Autodesk Fusion 360 part; units mm, degrees
sketch "Sketch1" plane through (0, 0, 0) normal (0, 0, 1) x (1, 0, 0)
  line L0 (-2.875, 0) -> (2.875, 0)
  line L1 (-5.375, 2.5) -> (5.375, 2.5)
  line L2 (-5.375, 2.5) -> (-2.875, 0)
  line L3 (5.375, 2.5) -> (2.875, 0)
  line L4 (0, 7.9451) -> (0, -6.0549)
  dimension "d1" = 5.75
  dimension "d2" = 10.75
  dimension "d3" = 2.5
extrude "Extrude1" add sketch "Sketch1" along normal blind 60
sketch "Sketch2" plane through (0, 0, 0) normal (0, 0, -1) x (-1, 0, 0)
  line L0 (2.875, 0) -> (5.375, 2.5)
  line L1 (5.375, 2.5) -> (-5.375, 2.5)
  line L2 (-5.375, 2.5) -> (-2.875, 0)
  line L3 (-2.875, 0) -> (2.875, 0)
  line L4 (-5.375, 2.5) -> (5.375, 2.5)
  line L5 (5.375, 2.5) -> (5.375, -3)
  line L6 (5.375, -3) -> (-5.375, -3)
  line L7 (-5.375, -3) -> (-5.375, 2.5)
  dimension "d6" = 10.75
  dimension "d7" = 5.5
extrude "Extrude2" add sketch "Sketch2" along normal blind 2.5
sketch "Sketch3" plane through (0, 0, 0) normal (0, -1, 0) x (1, 0, 0)
  line L0 (-2.875, 0) -> (2.875, 0)
  line L1 (2.875, 0) -> (2.875, 60)
  line L2 (2.875, 60) -> (-2.875, 60)
  line L3 (-2.875, 60) -> (-2.875, 0)
  circle A0 centre (0, 10) radius 1.5
  circle A1 centre (0, 30) radius 1.5
  circle A2 centre (0, 50) radius 1.5
  dimension "d10" = 3
  dimension "d11" = 10
  dimension "d12" = 30
  dimension "d13" = 20
extrude "Extrude3" cut sketch "Sketch3" against normal through all contours A0 | A1 | A2
The listing builds one solid part. Answer for the finished solid, in the listing's coordinates (mm). A direction names the side the tool comes from. Coordinates: 2 decimals unless noted, no trailing zeros. Order: outer loops, then holes, each group sorted by start corner. A loop starts at its lowest first (then second) coordinate and runs counter-clockwise, first axis right, second up. Notation, with made-up numbers: M 82,57 L 116,57 A27 cw 116,86 Z; hole C 23,6.25 d11. An arc over 180 degrees is marked long. Use CSV: the item, a comma, the result in double quotes.
Q1. Section A-A (x = 0) is taken. Determine the outline of the cut face in (y, z), then the cut area to 3 significant figures.
Here are the results:
outline,"M -3,-2.5 L 2.5,-2.5 L 2.5,8.5 L 0,8.5 L 0,0 L -3,0 Z; M 0,11.5 L 2.5,11.5 L 2.5,28.5 L 0,28.5 Z; M 0,31.5 L 2.5,31.5 L 2.5,48.5 L 0,48.5 Z; M 0,51.5 L 2.5,51.5 L 2.5,60 L 0,60 Z"
area,"141 mm2"
Q2. Section D-D (y = -1.9) is taken. Determine the outline of the cut face in (x, z) (3 decimals).
Here are the results:
outline,"M -5.375,-2.5 L 5.375,-2.5 L 5.375,0 L -5.375,0 Z"
Q3. Determine the mould class of faces 1 (the cylindrical face through (-0.195, 1.232, 31.487)), 2 (the flat face through (-2, 0, 30)), 3 (the flat face through (4.142, 1.267, 29.58)) for opening direction X: pulls with the +X half, pulls with the -X half, needs draft (parallel to the pull), parting line crosses it, or undercut.
Here are the results:
face 1,"undercut"
face 2,"needs draft"
face 3,"pulls with the +X half"
Q4. Section B-B (z = 50) is taken. Determine the outline of the cut face in (x, y) (3 decimals).
Here are the results:
outline,"M -5.375,2.5 L -2.875,0 L -1.5,0 L -1.5,2.5 Z; M 1.5,0 L 2.875,0 L 5.375,2.5 L 1.5,2.5 Z"
Q5. Given pin 1 Ø4 at (x, z) = (0, 30) entering from -Y, flat-ended and moving along its own axis, determine where the tip first touches the part or whether it passes through.
Here are the results:
pin 1,"y = 0"
Q6. Section C-C (y = 1.7) is taken. Determine the outline of the cut face in (x, z) (3 decimals), then the cut area to 3 significant figures.
Here are the results:
outline,"M -5.375,-2.5 L 5.375,-2.5 L 5.375,0 L 4.575,0 L 4.575,60 L -4.575,60 L -4.575,0 L -5.375,0 Z; hole C 0,10 d3; hole C 0,30 d3; hole C 0,50 d3"
area,"555 mm2"
Q7. A tool of negligible diameter and unlimited length cuts with its end or side. For faces 4 (the flat face through (-4.142, 1.267, 29.58)), 5 (the flat face through (5.375, 0, -1)), from which of +Z, -Z, +X, -X, +Y, -Y can it reach the whole face along a straight path? Write none if from no direction.
Here are the results:
face 4,"+Z, -X, -Y"
face 5,"+Z, -Z, +X, +Y, -Y"
Q8. Straight lines are drawn through the part: L1, parallel to Z at x = 0, y = 1.35; L2, parallel to Z at x = -0.5, y = -0.95; L3, parallel to Y at x = 2.25, z = 11.5. For each, find the intervals that lie inside material, in ascending order.
Here are the results:
L1,"-2.5 to 8.5, 11.5 to 28.5, 31.5 to 48.5, 51.5 to 60"
L2,"-2.5 to 0"
L3,"0 to 2.5"
